Autodesk Inventor part; units mm, degrees
ref_plane "YZ Plane" through (0, 0, 0) normal (1, 0, 0) x (0, 1, 0)
ref_plane "XZ Plane" through (0, 0, 0) normal (0, 1, 0) x (-1, 0, 0)
ref_plane "XY Plane" through (0, 0, 0) normal (0, 0, 1) x (1, 0, 0)
sketch "Sketch_1" plane through (0, 0, 0) normal (0, 0, 1) x (1, 0, 0)
  line L0 (4.5, 0) -> (-2.8, 0)
  line L1 (-2.8, 0) -> (-2.8, 5)
  line L2 (-2.8, 5) -> (0, 5)
  line L3 (0, 5) -> (0, 3)
  line L4 (0, 3) -> (4.5, 3)
  line L5 (4.5, 3) -> (4.5, 0)
  line L6 (4.5, 0) -> (-2.8, 0)
revolve "Revolution1" add sketch "Sketch_1" angle 360 about axis through (4.5, 0, 0) along (1, 0, 0)
sketch "Sketch2" plane through (-2.8, 0, 0) normal (-1, 0, 0) x (0, 0, 1)
  point P0 (0, 0)
hole "Hole1" at (-2.8, 0, 0) direction (1, 0, 0) diameter 2.5 depth 2.5 tip angle 120
sketch "Sketch_3" plane through (-2.8, 0, 0) normal (1, 0, 0) x (0, 0, -1)
  line L0 (-1.25, -0.7217) -> (0, -1.4434)
  line L1 (0, -1.4434) -> (1.25, -0.7217)
  line L2 (1.25, -0.7217) -> (1.25, 0.7217)
  line L3 (1.25, 0.7217) -> (0, 1.4434)
  line L4 (0, 1.4434) -> (-1.25, 0.7217)
  line L5 (-1.25, 0.7217) -> (-1.25, -0.7217)
extrude "Extrusion1" cut sketch "Sketch_3" along normal blind 2.5
sketch "Sketch_6" plane through (0, 0, 0) normal (0, 0, 1) x (1, 0, 0)
  line L0 (9.5, 0) -> (4.5, 0)
  line L1 (4.5, 0) -> (4.5, 2)
  line L2 (4.5, 2) -> (9.0705, 2)
  line L3 (9.0705, 2) -> (9.5, 1.5705)
  line L4 (9.5, 1.5705) -> (9.5, 0)
  line L5 (9.5, 0) -> (4.5, 0)
revolve "Revolution2" add sketch "Sketch_6" angle 360 about axis through (9.5, 0, 0) along (1, 0, 0)
thread "Thread1"
sketch "スケッチ5" plane through (9.5, 0, 0) normal (1, 0, 0) x (0, 0, -1)
  circle A0 centre (0, 0) radius 5
extrude "押し出し2" cut sketch "スケッチ5" against normal blind 2
properties part number "DBTS4-4_5-5-LTC_mod"
Model file for the job. Use its own axes, mm. A direction names the side the tool comes from. Coordinates: 2 decimals unless noted, no trailing zeros. Order: outer loops, then holes, each group sorted by start corner. A loop starts at its lowest first (then second) coordinate and runs counter-clockwise, first axis right, second up. Notation, with made-up numbers: (28.25, 37) -> (73.25, 37) arc R33 cw to (73.25, 73) -> close; hole circle Ø6 at (57, 6.25). An arc over 180 degrees is marked (long way). Answer as a JSON object with one key per item and string values. Group by question number.
1) Cut at C-C, the plane x = 6.5. Write the cut outline in (y, z).
2) Pull direction Y, two halves, no side cores. Call faces 1 (the face through (-2, 0, -1.25)), 2 (the face through (-1.38, -1.08, -4.88)), 3 (the face through (-1.57, -1.08, 0.63)), 4 (the face through (0, 3.3, 0.1)): +Y half, -Y half, draft (parallel to the pull), parting line (faces both ways), or undercut.
3) Cut at A-A, the plane x = -0.75. Write the cut outline in (y, z).
4) Drill centre lines: L1, parallel to X at y = 2.25, z = 1.25; L2, parallel to X at y = 3.5, z = -0.75; L3, parallel to Z at x = -1.25, y = -1. Where is each one in solid material? Low to high.
5) Which spindle directions (+Z, -Z, +X, -X, +Y, -Y) get a long thin tool onto all of the face, cutting with end or side? Do faces 5 (the face through (-2.8, 1.04, -1.04)), 6 (the face through (-2, 0, 1.25)), 7 (the face through (4.5, 1, -2)). Say none if no direction does.
6) Flat gauge pin, fed straight in: pin 1 (1 mm diameter, centred on x = 4, z = 0.5, fed in from +Y). Where does the tip first touch, or does it go through?
7) Cut at D-D, the plane y = 3.75. Write the cut outline in (x, z).
8) Cut at B-B, the plane z = -2.5. Write the cut outline in (x, y).
Check values:
{
 "1": {"outline": "circle Ø4 at (0, 0)"},
 "2": {"face 1": "undercut", "face 2": "parting line", "face 3": "undercut", "face 4": "draft"},
 "3": {"outline": "circle Ø10 at (0, 0); hole (-1.44, 0) -> (-0.72, -1.25) -> (0.72, -1.25) -> (1.44, 0) -> (0.72, 1.25) -> (-0.72, 1.25) -> close"},
 "4": {"L1": "x = -2.8 to 4.5", "L2": "x = -2.8 to 0", "L3": "z = -4.9 to -0.77, 0.77 to 4.9"},
 "5": {"face 5": "+Z, -Z, -X, +Y, -Y", "face 6": "-X", "face 7": "+X"},
 "6": {"pin 1": "stops at y = 3"},
 "7": {"outline": "(-2.8, -3.31) -> (0, -3.31) -> (0, 3.31) -> (-2.8, 3.31) -> close"},
 "8": {"outline": "(-2.8, -4.33) -> (0, -4.33) -> (0, -1.66) -> (4.5, -1.66) -> (4.5, 1.66) -> (0, 1.66) -> (0, 4.33) -> (-2.8, 4.33) -> close"}
}
